Autodesk Inventor part; units mm, degrees
ref_plane "YZ Plane" through (0, 0, 0) normal (1, 0, 0) x (0, 1, 0)
ref_plane "XZ Plane" through (0, 0, 0) normal (0, 1, 0) x (-1, 0, 0)
ref_plane "XY Plane" through (0, 0, 0) normal (0, 0, 1) x (1, 0, 0)
sketch "Sketch1" plane through (0, 0, 0) normal (0, 1, 0) x (-1, 0, 0)
  circle A0 centre (0, 0) radius 150
  line L0 (150, 0) -> (0, 0)
  line L1 (0, 0) -> (-75, -129.9038)
  line L2 (0, 0) -> (150, 0) construction
  line L3 (0, 0) -> (-75, 129.9038)
  line L4 (0, 0) -> (150, 0) construction
  line L5 (-75, 129.9038) -> (-74.5, 129.0378)
  line L6 (-74.5, 129.0378) -> (-69.335, 120.0917)
  line L7 (-75, 129.9038) -> (-64.967, 112.5261)
  circle A1 centre (-64.967, 112.5261) radius 1.5
  line L8 (150, 0) -> (129.934, 0)
  circle A2 centre (129.934, 0) radius 1.5
  line L9 (-75, -129.9038) -> (-64.967, -112.5261)
  circle A3 centre (-64.967, -112.5261) radius 1.5
  dimension "d20" = 300
  dimension "d22" = 120
  dimension "d23" = 120
  dimension "d24" = 1
  dimension "d25" = 10.33
  dimension "d26" = 20.066
  dimension "d27" = 3
  dimension "d28" = 20.066
  dimension "d29" = 3
  dimension "d30" = 20.066
  dimension "d31" = 3
extrude "Extrusion1" add sketch "Sketch1" along normal blind 6.35 contours L0 A2 L3 A1 A0 | A0 L1 A3 L0 A2 | L3 A1 L1 A3 A0
sketch "Sketch2" plane through (0, 6.35, 0) normal (0, 1, 0) x (1, 0, 0)
  circle A0 centre (-129.934, 0) radius 1.5
  line L0 (-129.934, -1.5) -> (-129.934, -11.5)
  line L1 (-129.934, 1.5) -> (-129.934, 11.5)
  circle A1 centre (-129.934, -11.5) radius 1.5
  circle A2 centre (-129.934, 11.5) radius 1.5
  circle A3 centre (64.967, -112.5261) radius 1.5
  line L2 (63.6961, -113.3229) -> (54.8713, -118.0264)
  line L3 (54.8713, -118.0264) -> (66.337, -111.9154)
  line L4 (66.337, -111.9154) -> (75.1618, -107.2119)
  circle A4 centre (54.8713, -118.0264) radius 1.5
  circle A5 centre (75.1618, -107.2119) radius 1.5
  circle A6 centre (64.967, 112.5261) radius 1.5
  line L5 (66.337, 111.9154) -> (74.3759, 105.9675)
  line L6 (74.3759, 105.9675) -> (63.9823, 113.6576)
  line L7 (63.9823, 113.6576) -> (55.9434, 119.6055)
  circle A7 centre (55.9434, 119.6055) radius 1.5
  circle A8 centre (74.3759, 105.9675) radius 1.5
  point P0 (0, 0)
  dimension "d36" = 10
  dimension "d37" = 10
  dimension "d38" = 3
  dimension "d39" = 3
  dimension "d40" = 10
  dimension "d41" = 10
  dimension "d42" = 3
  dimension "d43" = 3
  dimension "d44" = 10
  dimension "d45" = 10
  dimension "d46" = 3
  dimension "d47" = 3
extrude "Extrusion3" cut sketch "Sketch2" against normal through all contours A1 | A2 | A4 | A5 | A8 | A7
sketch "Sketch7" plane through (0, 6.35, 0) normal (0, 1, 0) x (1, 0, 0)
  circle A0 centre (0, 0) radius 150
  line L0 (150, 0) -> (-150, 0)
properties part number "plate support" material "Polycarbonat, klar"
Build history of the part. All positions in model axes, mm. Give positions to 0.01 mm unless a question says otherwise; leave off trailing zeros. Order: outer loops, then holes, each group sorted by start corner. A loop starts at its lowest first (then second) coordinate and runs counter-clockwise, first axis right, second up. Notation, with made-up numbers: M 83,-30.75 L 135,-30.75 A29 cw 135,-2.75 Z; hole C 53.5,68 d2. An arc over 180 degrees is marked long. Put each result on its own line as item: value.
Item 1: Slice it at C-C, the plane x = -109. Write the cut outline in (y, z).
From the geometry:
outline: M 0,-103.05 L 6.35,-103.05 L 6.35,103.05 L 0,103.05 Z
Item 2: Slice it at B-B, the plane z = -40. Write the cut outline in (x, y).
From the geometry:
outline: M -144.57,0 L 144.57,0 L 144.57,6.35 L -144.57,6.35 Z
Item 3: Flat gauge pins, fed straight in: pin 1 Ø4 at (x, z) = (64.97, 112.53) entering from -Y; pin 2 Ø1.5 at (y, z) = (1.5, 39) entering from +X; pin 3 Ø1 at (y, z) = (4.5, 118.5) entering from -X; pin 4 Ø2 at (y, z) = (2.5, -27.5) entering from -X. Where does each tip first touch, or does it go through?
From the geometry:
pin 1: stops at y = 0
pin 2: stops at x = 145.04
pin 3: stops at x = -92.61
pin 4: stops at x = -147.64
Item 4: Probe line 1 (X direction, y = 4.25, z = 0); line 2 (X direction, y = 3.25, z = -11.5); line 3 (Z direction, x = -42, y = 2). List the from-to ranges inside material, lowest first. Write a range as [from, to].
From the geometry:
line 1: x = [-150, -131.43], [-128.43, 150]
line 2: x = [-149.56, -131.43], [-128.43, 149.56]
line 3: z = [-144, 144]
Item 5: Slice it at A-A, the plane y = 4.25. Give the number of separate pieces and of enclosed holes in the cut face, plus the area to 3 significant figures.
From the geometry:
separate pieces: 1
enclosed holes: 9
area: 70,600 mm2
